Part model, mm, in its own coordinate system. Face numbers are marked on the shaded views. A direction names the side the tool comes from. Give positions to 0.01 mm unless a question says otherwise; leave off trailing zeros. Write each loop counter-clockwise with the first axis right and the second up, starting at its lowest first coordinate (ties: lowest second). Pieces come first, ordered by that corner, then holes. Notation, with made-up numbers: M -11.75,71 L 45.25,71 A18 cw 45.25,100 Z; hole C -2.75,72 d3. An arc over 180 degrees is marked long. Use a Markdown table: item, result.
Autodesk Inventor part; units mm, degrees
ref_plane "YZ Plane" through (0, 0, 0) normal (1, 0, 0) x (0, 1, 0)
ref_plane "XZ Plane" through (0, 0, 0) normal (0, 1, 0) x (-1, 0, 0)
ref_plane "XY Plane" through (0, 0, 0) normal (0, 0, 1) x (1, 0, 0)
sketch "Sketch1" plane through (0, 0, 0) normal (0, 1, 0) x (-1, 0, 0)
  line L0 (-20.5, 10.75) -> (20.5, 10.75)
  line L1 (20.5, 10.75) -> (20.5, -10.75)
  line L2 (20.5, -10.75) -> (-20.5, -10.75)
  line L3 (-20.5, -10.75) -> (-20.5, 10.75)
  line L4 (-20.5, 10.75) -> (20.5, -10.75) construction
  line L5 (20.5, 10.75) -> (-20.5, -10.75) construction
  line L6 (-24.25, 5) -> (24.25, 5) construction
  line L7 (24.25, 5) -> (24.25, -5) construction
  line L8 (24.25, -5) -> (-24.25, -5) construction
  line L9 (-24.25, -5) -> (-24.25, 5) construction
  line L10 (-24.25, 5) -> (24.25, -5) construction
  line L11 (24.25, 5) -> (-24.25, -5) construction
  circle A0 centre (24.25, 5) radius 2.75
  circle A1 centre (24.25, -5) radius 2.75
  circle A2 centre (-24.25, 5) radius 2.75
  circle A3 centre (-24.25, -5) radius 2.75
  line L12 (30.25, 9.75) -> (30.25, -9.75)
  line L13 (25.25, -14.75) -> (0, -14.75)
  line L14 (25.25, 14.75) -> (0, 14.75)
  line L15 (0, 14.75) -> (0, 0) construction
  line L16 (0, 0) -> (0, -14.75) construction
  arc A4 (30.25, 9.75) -> (25.25, 14.75) centre (25.25, 9.75) ccw
  arc A5 (25.25, -14.75) -> (30.25, -9.75) centre (25.25, -9.75) ccw
  line L17 (20.5, 2.5) -> (20.5, 2.5)
  line L18 (22.5, 0.5) -> (22.5, -0.5)
  line L19 (20.5, -2.5) -> (20.5, -2.5)
  line L20 (20.5, -2.5) -> (20.5, 2.5)
  line L21 (20.5, 2.5) -> (22.5, -2.5) construction
  line L22 (22.5, 2.5) -> (20.5, -2.5) construction
  line L23 (21.5, 0) -> (0, 0) construction
  line L24 (-30.25, 9.75) -> (-30.25, -9.75)
  line L25 (-25.25, -14.75) -> (0, -14.75)
  line L26 (-25.25, 14.75) -> (0, 14.75)
  arc A6 (-25.25, 14.75) -> (-30.25, 9.75) centre (-25.25, 9.75) ccw
  arc A7 (-30.25, -9.75) -> (-25.25, -14.75) centre (-25.25, -9.75) ccw
  arc A8 (22.5, 0.5) -> (20.5, 2.5) centre (20.5, 0.5) ccw
  arc A9 (20.5, -2.5) -> (22.5, -0.5) centre (20.5, -0.5) ccw
  line L27 (-20.5, 2.5) -> (-20.5, 2.5)
  line L28 (-22.5, 0.5) -> (-22.5, -0.5)
  line L29 (-20.5, -2.5) -> (-20.5, -2.5)
  line L30 (-20.5, -2.5) -> (-20.5, 2.5)
  line L31 (-20.5, 2.5) -> (-22.5, -2.5) construction
  line L32 (-22.5, 2.5) -> (-20.5, -2.5) construction
  arc A10 (-20.5, 2.5) -> (-22.5, 0.5) centre (-20.5, 0.5) ccw
  arc A11 (-22.5, -0.5) -> (-20.5, -2.5) centre (-20.5, -0.5) ccw
  point P0 (20.5, 2.5)
  point P1 (20.5, -2.5)
  point P2 (-21.5, 0)
  point P3 (-20.5, -2.5)
  point P4 (-20.5, 2.5)
  point P5 (20.5, 3.5)
  point P6 (20.5, -3.5)
  point P7 (-20.5, -3.5)
  point P8 (-20.5, 3.5)
  dimension "d0" = 21.5
  dimension "d1" = 41
  dimension "d2" = 5.5
  dimension "d3" = 48.5
  dimension "d4" = 10
  dimension "d5" = 4
  dimension "d6" = 4
  dimension "d7" = 6
  dimension "d8" = 5
  dimension "d9" = 5
  dimension "d10" = 5
  dimension "d11" = 2
  dimension "d12" = 2
extrude "Extrusion1" add sketch "Sketch1" along normal blind 8.5 contours L3 A11 L28 A10 | L12 A5 L13 L25 A7 L24 A6 L26 L14 A4
sketch "Sketch2" plane through (-25.25, 0, 14.75) normal (0, 0, 1) x (1, 0, 0)
  line L0 (0, 8.5) -> (50.5, 8.5) construction
  line L1 (7.25, 8.5) -> (13.8046, 3)
  line L2 (13.8046, 3) -> (25.25, 3)
  line L3 (25.25, 3) -> (25.25, 8.5)
  line L4 (7.25, 8.5) -> (25.25, 8.5)
  line L5 (43.25, 8.5) -> (36.6954, 3)
  line L6 (36.6954, 3) -> (25.25, 3)
  line L7 (43.25, 8.5) -> (25.25, 8.5)
  point P0 (25.25, 0)
  dimension "d15" = 18
  dimension "d16" = 40
  dimension "d17" = 3
extrude "Extrusion2" cut sketch "Sketch2" against normal through all
fillet "Fillet1" radius 2 2 edges at (-20.5, 4.25, 2.5) (-20.5, 4.25, -2.5)
equation "\"d6\" = d5"
properties part number "CH_01_0035_servo_mount" material "Acetal Resin, Black"
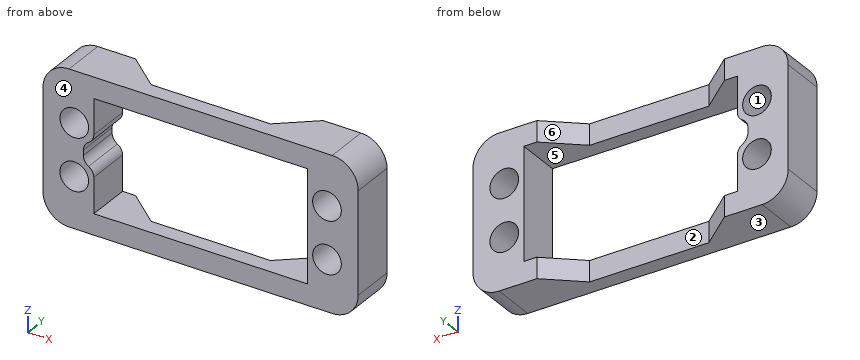
1. Cut at B-B, the plane z = 5. Give the cut face in (x, y).
Findings below:
| item | result |
|---|---|
| outline | M -30.25,0 L -27,0 L -27,8.5 L -30.25,8.5 Z; M -21.5,0 L -20.5,0 L -20.5,8.5 L -21.5,8.5 Z; M 20.5,0 L 21.5,0 L 21.5,8.5 L 20.5,8.5 Z; M 27,0 L 30.25,0 L 30.25,8.5 L 27,8.5 Z |
2. Tool access for the marked faces 4, 5 and 6: list every direction of +Z, -Z, +X, -X, +Y, -Y with a clear straight run to the whole face (end or side of a thin tool).
Findings below:
| item | result |
|---|---|
| face 4 | +Z, -Z, +X, -X, -Y |
| face 5 | +Y, -Y |
| face 6 | +Z, -Z, +Y |
3. Two-plate mould, pull along Z, no slides. Class the marked faces 1, 2 and 3: released by +Z, released by -Z, zero draft, split by the parting line, or undercut.
Findings below:
| item | result |
|---|---|
| face 1 | undercut |
| face 2 | zero draft |
| face 3 | released by -Z |
4. Cut at D-D, the plane y = 4. State how many separate pieces and enclosed holes the cut face has, then the cut area to 3 significant figures.
Findings below:
| item | result |
|---|---|
| separate pieces | 2 |
| enclosed holes | 4 |
| area | 576 mm2 |
5. Drop a flat-ended pin along its axis: P1, Ø3, axis at x = -3.5, z = 12.5, coming from the +Y side. Give the stop position or say it passes through.
Findings below:
| item | result |
|---|---|
| P1 | y = 3 |
6. Drill centre lines: L1, parallel to Z at x = -24.25, y = 4.25; L2, parallel to Z at x = -4, y = 2.25; L3, parallel to X at y = 4.25, z = 4. Where is each one in solid material? Low to high.
Findings below:
| item | result |
|---|---|
| L1 | -14.75 to -7.75, -2.25 to 2.25, 7.75 to 14.75 |
| L2 | -14.75 to -10.75, 10.75 to 14.75 |
| L3 | -30.25 to -26.81, -21.69 to -20.5, 20.5 to 21.69, 26.81 to 30.25 |
7. Cut at C-C, the plane x = 24.25. Give the cut face in (y, z).
Findings below:
| item | result |
|---|---|
| outline | M 0,-14.75 L 8.5,-14.75 L 8.5,-7.75 L 0,-7.75 Z; M 0,-2.25 L 8.5,-2.25 L 8.5,2.25 L 0,2.25 Z; M 0,7.75 L 8.5,7.75 L 8.5,14.75 L 0,14.75 Z |
8. Cut at A-A, the plane y = 1.5. Give the cut face in (x, z), then the cut area to 3 significant figures.
Findings below:
| item | result |
|---|---|
| outline | M -30.25,-9.75 A5 ccw -25.25,-14.75 L 25.25,-14.75 A5 ccw 30.25,-9.75 L 30.25,9.75 A5 ccw 25.25,14.75 L -25.25,14.75 A5 ccw -30.25,9.75 Z; hole C -24.25,-5 d5.5; hole C -24.25,5 d5.5; hole M -22.5,-0.5 A2 ccw -21.5,-2.23 A2 cw -20.5,-3.96 L -20.5,-10.75 L 20.5,-10.75 L 20.5,10.75 L -20.5,10.75 L -20.5,3.96 A2 cw -21.5,2.23 A2 ccw -22.5,0.5 Z; hole C 24.25,-5 d5.5; hole C 24.25,5 d5.5 |
| area | 778 mm2 |
